Input: part model. Units: mm. Frame: model coordinates. A direction names the side the tool comes from. Round coordinates to 2 decimals unless told otherwise and drop trailing zeros. Loops run counter-clockwise (first coordinate to the right, second up) from the corner with the lowest first, then second, coordinate; pieces in that order, holes last.
1) Section C-C, the plane z = 7.5. Return loops of the section in (x, y) (3 decimals), and give its area (3 significant figures).
2) Draft query along X for faces 4 (the face through (87.284, 18, 5)), 5 (the face through (48, 19.93, 5)), 6 (the face through (5, 2, 5)). Return one class per face: pulls with the +X half, pulls with the -X half, needs draft (parallel to the pull), parting line crosses it, or undercut.
3) Section D-D, the plane x = 68. Return loops of the section in (y, z), and give its area (3 significant figures).
4) Section A-A, the plane x = 0. Return loops of the section in (y, z), and give its area (3 significant figures).
5) Ray query, line 1 along Y through (x, z) = (0, 3); line 2 along X through (y, z) = (0, 4.75); line 3 along Y through (x, z) = (66, 2.25). Return the intervals inside material, ascending.
6) Section B-B, the plane y = 0. Return loops of the section in (x, z), and give its area (3 significant figures).
7) First-contact query: pin 1 (3 mm diameter, centred on x = 42.5, z = 3, fed in from -Y); pin 2 (4 mm diameter, centred on x = 6.5, z = 6, fed in from -Y); pin 3 (3 mm diameter, centred on y = 7.5, z = 2.5, fed in from +X). Flat tips, straight axial feed; report the tip coordinate or a pass-through.
8) Access query for faces 1 (the face through (7, -2.013, 5)), 2 (the face through (31, 17, 9.398)), 3 (the face through (-1.321, 0, 5)). Directions: +Z, -Z, +X, -X, +Y, -Y. A direction counts if a zero-diameter tool reaches every point of the face in a straight line with its end or side. Return the directions, or none.
Autodesk Inventor part; units mm, degrees
ref_plane "YZ Plane" through (0, 0, 0) normal (1, 0, 0) x (0, 1, 0)
ref_plane "XZ Plane" through (0, 0, 0) normal (0, 1, 0) x (-1, 0, 0)
ref_plane "XY Plane" through (0, 0, 0) normal (0, 0, 1) x (1, 0, 0)
sketch "Sketch2" plane through (0, 0, 0) normal (0, 0, 1) x (1, 0, 0)
  circle A0 centre (0, 0) radius 2
  circle A1 centre (0, 0) radius 4
  line L0 (3.4641, 2) -> (6.0041, 2)
  line L1 (6.0041, 2) -> (6.0041, -2.0132)
  line L2 (6.0041, -2.0132) -> (3.4564, -2.0132)
  line L3 (-1.3208, -1.5018) -> (-1.3208, 1.5018)
  dimension "d7" = 4
  dimension "d8" = 8
  dimension "d9" = 2.54
  dimension "d10" = 4.0132
  dimension "d11" = 2
  dimension "d25" = 1.3208
extrude "Extrusion2" add sketch "Sketch2" along normal blind 9.398
sketch "Sketch3" plane through (6.0041, -2.0132, 0) normal (1, 0, 0) x (0, 0, -1)
  line L0 (-9.398, 0) -> (-9.398, 4.0132)
  line L1 (-9.398, 4.0132) -> (-9.398, 0)
  line L2 (-9.398, 0) -> (0, 0)
  line L3 (0, 0) -> (0, 4.0132)
  line L4 (0, 0) -> (0, 4.0132)
  line L5 (0, 4.0132) -> (-9.398, 4.0132)
  line L6 (0, 4.0132) -> (-9.398, 4.0132)
  point P0 (0, 2.0132)
extrude "Extrusion3" add sketch "Sketch3" along normal blind 5.08
sketch "Sketch4" plane through (3.4641, 2, 9.398) normal (0, 1, 0) x (1, 0, 0)
  line L0 (0, 0) -> (7.62, 0)
  line L1 (7.62, 0) -> (3.81, 0)
  line L2 (3.81, 0) -> (3.81, 9.398)
  line L3 (3.81, 9.398) -> (7.62, 9.398)
  line L4 (7.62, 9.398) -> (7.62, 0)
  point P0 (-3.4641, 9.398)
  dimension "d16" = 3.81
  dimension "d17" = 9.398
extrude "Extrusion4" add sketch "Sketch4" along normal blind 17.9303
sketch "Sketch5" plane through (11.0841, -2.0132, 0) normal (1, 0, 0) x (0, 0, -1)
  line L0 (0, 21.9435) -> (0, 18.04)
  line L1 (0, 18.04) -> (-9.398, 18.04)
  line L2 (-9.398, 18.04) -> (-9.398, 21.9435)
  line L3 (0, 0) -> (0, 21.9435)
  line L4 (-9.398, 21.9435) -> (0, 21.9435)
  point P0 (0, 2.0132)
  point P1 (-9.398, 21.9435)
  dimension "d29" = 9.398
  dimension "d30" = 3.9035
  dimension "d31" = 3.9035
extrude "Extrusion5" add sketch "Sketch5" along normal blind 76.2
fillet "Fillet1" radius 3.175 1 edges at (7.2741, 19.9303, 4.699)
fillet "Fillet2" radius 3.175 1 edges at (11.0841, 16.0268, 4.699)
sketch "Sketch6" plane through (0, 0, 9.398) normal (0, 0, 1) x (1, 0, 0)
  circle A0 centre (0, 0) radius 2
  line L0 (-1.3208, -1.5018) -> (-1.3208, 1.5018)
  arc A1 (-1.3208, 1.5018) -> (-1.3208, -1.5018) centre (0, 0) ccw
  dimension "d26" = 1.3208
extrude "Extrusion6" add sketch "Sketch6" against normal blind 9.398 contours L0 A0 picked at (-1.5423, 0.0807)
properties part number "Rotator"
Final values:
1. outline: (3.456, -2.013) - (11.084, -2.013) - (11.084, 12.852) arc R3.175 cw to (14.259, 16.027) - (87.284, 16.027) - (87.284, 19.93) - (10.449, 19.93) arc R3.175 ccw to (7.274, 16.755) - (7.274, 2) - (3.464, 2) arc R4 ccw (long way) to start; hole (-1.321, -1.502) arc R2 ccw (long way) to (-1.321, 1.502) - close
1. area: 434 mm2
2. face 4: pulls with the +X half
2. face 5: needs draft
2. face 6: undercut
3. outline: (16.03, 0) - (19.93, 0) - (19.93, 9.4) - (16.03, 9.4) - close
3. area: 36.7 mm2
4. outline: (-4, 0) - (-2, 0) - (-2, 9.4) - (-4, 9.4) - close; (2, 0) - (4, 0) - (4, 9.4) - (2, 9.4) - close
4. area: 37.6 mm2
5. line 1: y = -4 to -2, 2 to 4
5. line 2: x = -4 to -1.32, 2 to 11.08
5. line 3: y = 16.03 to 19.93
6. outline: (-4, 0) - (-1.32, 0) - (-1.32, 9.4) - (-4, 9.4) - close; (2, 0) - (11.08, 0) - (11.08, 9.4) - (2, 9.4) - close
6. area: 111 mm2
7. pin 1: stops at y = 16.03
7. pin 2: stops at y = -2.01
7. pin 3: stops at x = 11.08
8. face 1: +Z, -Z, +X, -Y
8. face 2: +Z, +X, -X, +Y, -Y
8. face 3: +Z, -Z
